```python
from build123d import *

# Parameters (mm, degrees)
BOSS_EXTRUDE1_DEPTH     = 13.1572
BOSS_EXTRUDE2_DEPTH     = 8.89
SKETCH3_W               = 66.04
SKETCH3_H               = 20.285187831
BOSS_EXTRUDE3_DEPTH     = 5.08
BOSS_EXTRUDE4_DEPTH     = 8.89
CUT_EXTRUDE1_DEPTH      = 64.71104446
CUT_EXTRUDE1_DEPTH_BACK = 64.71104446
SKETCH6_R               = 5.1435
SKETCH7_W               = 66.04
SKETCH7_H               = 20.285187831
BOSS_EXTRUDE5_DEPTH     = 25.4
SKETCH9_W               = 1.615391333
SKETCH9_H               = 12.791830428
BOSS_EXTRUDE6_DEPTH     = 19.05
SKETCH10_R              = 5.08
CUT_EXTRUDE2_DEPTH      = 15.24
CUT_EXTRUDE3_DEPTH      = 1.27
SKETCH14_W              = 1.4732
SKETCH14_H              = 13.1572
CUT_EXTRUDE4_DEPTH      = 15.24
SKETCH15_W              = 64.77
SKETCH15_H              = 20.285187831
CUT_EXTRUDE5_DEPTH      = 19.05
BOSS_EXTRUDE7_DEPTH     = 1.4986
SKETCH17_W              = 64.77
SKETCH17_H              = 42.3672
CUT_EXTRUDE7_DEPTH      = 6.35


with BuildPart() as part:
    # Sketch1 → Boss-Extrude1 (new body)
    with BuildSketch(Plane(origin=(0, 0, 0), x_dir=(1, 0, 0), z_dir=(0, 1, 0))):
        Polygon((3.949839476, 3.210057439), (3.949839476, 17.1069), (0, 17.1069), (0, 0), (0, -3.178287831), (66.04, -3.178287831), (66.04, 0), (66.04, 17.1069), (62.090160524, 17.1069), (62.090160524, 3.210057439), (60.616960524, 3.210057439), (60.616960524, 17.1069), (55.050578368, 17.1069), (55.050578368, 3.210057439), (55.050578368, 0), (10.989421632, 0), (10.989421632, 3.210057439), (10.989421632, 17.1069), (5.423039476, 17.1069), (5.423039476, 3.210057439), align=None)
    extrude(amount=BOSS_EXTRUDE1_DEPTH)

    # Sketch2 → Boss-Extrude2 (add)
    with BuildSketch(Plane(origin=(0, 13.1572, 0), x_dir=(1, 0, 0), z_dir=(0, 1, 0))):
        Polygon((10.989421632, 17.1069), (0, 17.1069), (0, -3.178287831), (66.04, -3.178287831), (66.04, 17.1069), (55.050578368, 17.1069), (55.050578368, -0.226283794), (10.989421632, 0), align=None)
    extrude(amount=BOSS_EXTRUDE2_DEPTH)

    # Sketch3 → Boss-Extrude3 (add)
    with BuildSketch(Plane(origin=(0, 22.0472, 0), x_dir=(1, 0, 0), z_dir=(0, 1, 0))):
        with Locations((33.02, 6.964306084)):
            Rectangle(SKETCH3_W, SKETCH3_H)
    extrude(amount=BOSS_EXTRUDE3_DEPTH)

    # Sketch4 → Boss-Extrude4 (add)
    with BuildSketch(Plane.XZ):
        Polygon((66.04, -17.1069), (55.050578368, -17.1069), (55.050578368, 0), (10.989421632, 0), (10.989421632, -17.1069), (0, -17.1069), (0, 3.178287831), (66.04, 3.178287831), align=None)
    extrude(amount=BOSS_EXTRUDE4_DEPTH)

    # Sketch6 → Cut-Extrude1 (cut, two sides: drawn at the far end of the back side and taken through both)
    with BuildSketch(Plane.ZY.offset(-55.050578368).offset(-CUT_EXTRUDE1_DEPTH_BACK)):
        with Locations((-17.1069, 6.5786)):
            Circle(SKETCH6_R)
    extrude(amount=CUT_EXTRUDE1_DEPTH + CUT_EXTRUDE1_DEPTH_BACK, mode=Mode.SUBTRACT)

    # Sketch7 → Boss-Extrude5 (add)
    with BuildSketch(Plane.XZ.offset(8.89)):
        with Locations((33.02, -6.964306084)):
            Rectangle(SKETCH7_W, SKETCH7_H)
    extrude(amount=BOSS_EXTRUDE5_DEPTH)

    # Sketch9 → Boss-Extrude6 (add)
    with BuildSketch(Plane(origin=(0, 0, -17.1069), x_dir=(-1, 0, 0), z_dir=(0, 0, -1))):
        Polygon((-41.375896334, 22.0472), (-41.18906329, 13.1572), (-40.971249817, 0.333691876), (-40.971249817, -8.89), (-37.490871957, -8.89), (-35.458871957, -8.89), (-35.458871957, 13.1572), (-35.458871957, 22.0472), align=None)
        with Locations((-38.298567624, 6.761284786)):
            Rectangle(SKETCH9_W, SKETCH9_H, mode=Mode.SUBTRACT)
    extrude(amount=-BOSS_EXTRUDE6_DEPTH)

    # Sketch10 → Cut-Extrude2 (cut)
    with BuildSketch(Plane.ZY.offset(-35.458871957)):
        with Locations((-17.1069, 6.5786)):
            Circle(SKETCH10_R)
    extrude(amount=-CUT_EXTRUDE2_DEPTH, mode=Mode.SUBTRACT)

    # Sketch12 → Cut-Extrude3 (cut)
    with BuildSketch(Plane(origin=(66.04, 0, 0), x_dir=(0, 0, -1), z_dir=(1, 0, 0))):
        Polygon((17.1069, 27.1272), (17.1069, 11.7221), (17.1069, 1.4351), (17.1069, -34.29), (-3.178287831, -34.29), (-3.52610715, 27.1272), align=None)
    extrude(amount=-CUT_EXTRUDE3_DEPTH, mode=Mode.SUBTRACT)

    # Sketch14 → Cut-Extrude4 (cut)
    with BuildSketch(Plane(origin=(0, 0, -17.1069), x_dir=(-1, 0, 0), z_dir=(0, 0, -1))):
        with Locations((-4.686439476, 6.5786)):
            Rectangle(SKETCH14_W, SKETCH14_H)
        with Locations((-1.511439476, 6.5786)):
            Rectangle(SKETCH14_W, SKETCH14_H)
    extrude(amount=-CUT_EXTRUDE4_DEPTH, mode=Mode.SUBTRACT)

    # Sketch15 → Cut-Extrude5 (cut)
    with BuildSketch(Plane.XZ.offset(34.29)):
        with Locations((32.385, -6.964306084)):
            Rectangle(SKETCH15_W, SKETCH15_H)
    extrude(amount=-CUT_EXTRUDE5_DEPTH, mode=Mode.SUBTRACT)

    # Sketch16 → Boss-Extrude7 (add)
    with BuildSketch(Plane.ZY.offset(-5.423039476)):
        with BuildLine():
            Line((-17.1069, 13.1572), (6.075816752, 13.1572))
            Line((6.075816752, 13.1572), (6.075816752, 0))
            Line((6.075816752, 0), (-17.1069, 0))
            Line((-17.1069, 0), (-17.1069, 1.4351))
            ThreePointArc((-17.1069, 1.4351), (-11.9634, 6.5786), (-17.1069, 11.7221))
            Line((-17.1069, 11.7221), (-17.1069, 13.1572))
        make_face()
    extrude(amount=BOSS_EXTRUDE7_DEPTH)

    # Sketch17 → Cut-Extrude7 (cut)
    with BuildSketch(Plane.XY.offset(3.178287831)):
        with Locations((32.385, 5.9436)):
            Rectangle(SKETCH17_W, SKETCH17_H)
    extrude(amount=-CUT_EXTRUDE7_DEPTH, mode=Mode.SUBTRACT)


with BuildPart() as body_2:
    # of the pieces the cut leaves, the one that is kept (cut_extrude7_keep)
    add(part.part.solids().sort_by_distance((10.989421632, 11.7221, -17.1069))[0])


solid = body_2.part
```
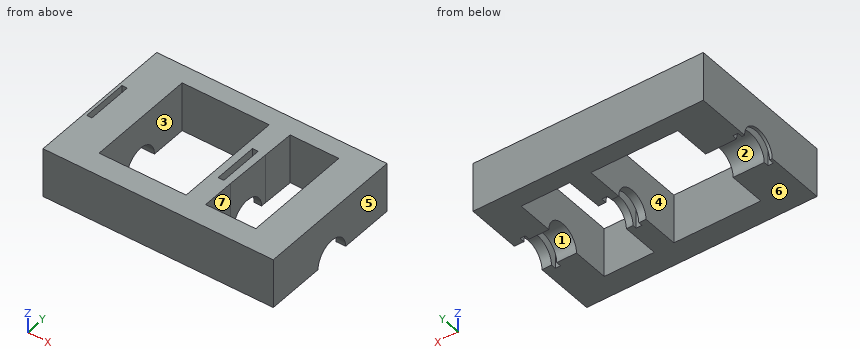
The listing builds one solid part. Answer for the finished solid, in the listing's coordinates (mm). Face numbers are marked on the shaded views. A direction names the side the tool comes from. Coordinates: 2 decimals unless noted, no trailing zeros. Write each loop counter-clockwise with the first axis right and the second up, starting at its lowest first coordinate (ties: lowest second). Pieces come first, ordered by that corner, then holes. Notation, with made-up numbers: (68.5, 15) - (78.5, 15) arc R27 cw to (78.5, 51) - close; hole circle Ø2 at (47.25, 17.25). An arc over 180 degrees is marked (long way). Return JSON: item names as keys, results as strings. Group by question number.
1. A cutting plane is placed at A-A, the plane y = -8. Determine the outline of the cut face in (x, z).
2. Which of the six approach directions +Z, -Z, +X, -X, +Y, -Y give full straight-line access (tool end or side, diameter ignored) to the marked faces 1, 2 and 3?
3. A cutting plane is placed at C-C, the plane z = -7. Determine the outline of the cut face in (x, y).
4. Straight lines are drawn through the part: L1, parallel to X at y = 1, z = -8; L2, parallel to X at y = -8, z = -13.25; L3, parallel to X at y = 12, z = -12.75. For each, find the intervals that lie inside material, in ascending order.
5. Given pin 1 (1.6 mm diameter, centred on x = 61, y = 3.5, fed in from -Z); pin 2 (5 mm diameter, centred on x = 34.5, y = 5, fed in from -Z), each flat-ended and moving along its own axis, determine where each tip first touches the part or whether it passes through.
6. Determine the mould class of the marked faces 4, 5, 6 and 7 for opening direction X: released by +X, released by -X, zero draft, split by the parting line, or undercut.
7. A cutting plane is placed at B-B, the plane x = 25. Determine the outline of the cut face in (y, z), plus the area to 3 significant figures.
8. A cutting plane is placed at D-D, the plane y = 17. Determine the outline of the cut face in (x, z), plus the area to 3 significant figures.
Ans:
{
 "1": {"outline": "(0, -17.11) - (10.99, -17.11) - (10.99, -3.17) - (0, -3.17) - close; (35.46, -17.11) - (40.97, -17.11) - (40.97, -3.17) - (35.46, -3.17) - close; (55.05, -17.11) - (64.77, -17.11) - (64.77, -3.17) - (55.05, -3.17) - close"},
 "2": {"face 1": "-Z, +X", "face 2": "-Z, -X", "face 3": "+Z, -Z"},
 "3": {"outline": "(0, -15.24) - (64.77, -15.24) - (64.77, 27.13) - (0, 27.13) - close; hole (0.77, 0) - (2.25, 0) - (2.25, 13.16) - (0.77, 13.16) - close; hole (10.99, -8.89) - (35.46, -8.89) - (35.46, 22.05) - (10.99, 22.05) - close; hole (37.49, 0.37) - (39.11, 0.37) - (39.11, 13.16) - (37.49, 13.16) - close; hole (40.97, -8.89) - (55.05, -8.89) - (55.05, 22.05) - (41.38, 22.05) - (41.19, 13.16) - (40.97, 0.33) - close; hole (60.62, 0) - (62.09, 0) - (62.09, 13.16) - (60.62, 13.16) - close"},
 "4": {"L1": "0 to 0.77, 2.25 to 10.99, 35.46 to 37.49, 39.11 to 40.98, 55.05 to 60.62, 62.09 to 64.77", "L2": "0 to 10.99, 35.46 to 40.97, 55.05 to 64.77", "L3": "0 to 0.77, 2.25 to 10.99, 35.46 to 37.49, 39.11 to 41.17, 55.05 to 60.62, 62.09 to 64.77"},
 "5": {"pin 1": "z = -13.62", "pin 2": "z = -13.84"},
 "6": {"face 4": "undercut", "face 5": "released by +X", "face 6": "zero draft", "face 7": "undercut"},
 "7": {"outline": "(-15.24, -17.11) - (-8.89, -17.11) - (-8.89, -3.17) - (-15.24, -3.17) - close; (22.05, -17.11) - (27.13, -17.11) - (27.13, -3.17) - (22.05, -3.17) - close", "area": "159 mm²"},
 "8": {"outline": "(0, -17.11) - (10.99, -17.11) - (10.99, -3.17) - (0, -3.17) - close; (35.46, -17.11) - (41.27, -17.11) - (41.27, -3.17) - (35.46, -3.17) - close; (55.05, -17.11) - (64.77, -17.11) - (64.77, -3.17) - (55.05, -3.17) - close", "area": "370 mm²"}
}
